```python
from build123d import *

# Parameters (mm, degrees)
SKETCH2_R                       = 1.875
BOSS_EXTRUDE1_DEPTH             = 10
BOSS_EXTRUDE1_DIRECTION_2_REACH = 9.5
SKETCH5_R                       = 1
CUT_EXTRUDE1_DEPTH              = 10


with BuildPart() as part:
    # Sketch1 → Revolve1 (revolve)
    with BuildSketch(Plane.XY):
        with BuildLine():
            Line((-3.247595264, -1.875), (-2.165063509, -1.25))
            ThreePointArc((-2.165063509, -1.25), (-2.165063509, 1.25), (0, 2.5))
            Line((0, 2.5), (0, 3.75))
            ThreePointArc((0, 3.75), (-3.247595264, 1.875), (-3.247595264, -1.875))
        make_face()
    revolve(axis=Axis((0, 2.5, 0), (0, 1, 0)))

    # Sketch2 → Boss-Extrude1 (add)
    with BuildSketch(Plane.XY.offset(3.75)):
        Circle(SKETCH2_R)
    extrude(amount=BOSS_EXTRUDE1_DEPTH)

    # Sketch2 → Boss-Extrude1 direction 2 (add, up to next)
    with BuildSketch(Plane.XY.offset(3.75), mode=Mode.PRIVATE) as boss_extrude1_direction_2_sk1:
        Circle(SKETCH2_R)
    boss_extrude1_direction_2_tool1 = extrude(boss_extrude1_direction_2_sk1.sketch, amount=-BOSS_EXTRUDE1_DIRECTION_2_REACH, mode=Mode.PRIVATE) - part.part
    add(boss_extrude1_direction_2_tool1.solids().sort_by_distance((0, 0, 3.75))[0])

    # Sketch5 → Cut-Extrude1 (cut)
    with BuildSketch(Plane.XY.offset(13.75)):
        Circle(SKETCH5_R)
    extrude(amount=-CUT_EXTRUDE1_DEPTH, mode=Mode.SUBTRACT)


solid = part.part
```
Design review of the part built by this model. Coordinates are the model's own, in mm. A direction names the side the tool comes from. Round coordinates to 2 decimals unless told otherwise and drop trailing zeros. Write each loop counter-clockwise with the first axis right and the second up, starting at its lowest first coordinate (ties: lowest second). Pieces come first, ordered by that corner, then holes.
Item 1: For faces 1 (the cylindrical face through (0, -1, 9)), 2 (the flat face through (1, -1, 13.75)), list the 3-axis set-ups (+Z, -Z, +X, -X, +Y, -Y) from which the entire face can be reached by the end or side of a thin tool; tool diameter is ignored.
Item 2: We need section D-D on z = 0. Write out the cut boundary in (x, y) (3 decimals), and give its area (3 significant figures).
Item 3: Clearance check with flat-ended pins moving along their axes: pin 1 Ø2 at (y, z) = (2.5, 4) entering from -X (3 decimals); pin 2 Ø2 at (x, y) = (2.5, 0) entering from -Z; pin 3 Ø1 at (y, z) = (0, 1.5) entering from -X. State where each tip first meets the part, or that it passes through.
Item 4: We need section C-C on y = 0.7. Write out the cut boundary in (x, z), and give its area (3 significant figures).
Item 5: We need section A-A on y = 0. Write out the cut boundary in (x, z) (3 decimals), and give its area (3 significant figures).
Item 6: We need section B-B on z = 11.25. Write out the cut boundary in (x, y) (3 decimals).
Item 7: For probe 1 along Y at (x, z) = (0, 9) (3 decimals); probe 2 along Z at (x, y) = (1, 0.7); probe 3 along Z at (x, y) = (-0.5, -0.35), list the stretches that pass through material, from the lowest coordinate up.
Returned:
1. face 1: +Z
1. face 2: +Z, +X, -X, +Y, -Y
2. outline: (-3.248, -1.875) - (-2.165, -1.25) arc R2.5 cw (long way) to (2.165, -1.25) - (3.248, -1.875) arc R3.75 ccw (long way) to start
2. area: 16.4 mm2
3. pin 1: stops at x = -1.125
3. pin 2: stops at z = -3.44
3. pin 3: stops at x = -3.61
4. outline: (-1.74, 3.25) arc R3.68 ccw (long way) to (1.74, 3.25) - (1.74, 13.75) - (0.71, 13.75) - (0.71, 3.75) - (-0.71, 3.75) - (-0.71, 13.75) - (-1.74, 13.75) - close; hole circle Ø4.8 at (0, 0)
4. area: 45.8 mm2
5. outline: (-1.875, 3.248) arc R3.75 ccw (long way) to (1.875, 3.248) - (1.875, 13.75) - (1, 13.75) - (1, 3.75) - (-1, 3.75) - (-1, 13.75) - (-1.875, 13.75) - close; hole circle Ø5 at (0, 0)
5. area: 42.7 mm2
6. outline: circle Ø3.75 at (0, 0); hole circle Ø2 at (0, 0)
7. probe 1: y = -1.875 to -1, 1 to 1.875
7. probe 2: z = -3.55 to -2.18, 2.18 to 13.75
7. probe 3: z = -3.7 to -2.42, 2.42 to 3.75
